Design review of the part built by this model. Coordinates are the model's own, in mm. A direction names the side the tool comes from. Coordinates: 2 decimals unless noted, no trailing zeros. Write each loop counter-clockwise with the first axis right and the second up, starting at its lowest first coordinate (ties: lowest second). Pieces come first, ordered by that corner, then holes. Notation, with made-up numbers: M 20.25,4 L 27.25,4 A26 cw 27.25,28 Z; hole C 72.5,-12.75 d10. An arc over 180 degrees is marked long. Return JSON: item names as keys, results as strings. Group by question number.
```python
from build123d import *

# Parameters (mm, degrees)
F0_R     = 2.25
F0_R_2   = 4
F1_DEPTH = 1.5


with BuildPart() as f1:
    # F0 (on Top) → F1 (new body)
    with BuildSketch(Plane.XY):
        Polygon((-7.522005, 11.843878), (-49.622005, 11.843878), (-49.622005, -3.456122), (-7.522005, -3.456122), (4.677995, -10.218692), (11.677995, -10.218692), (11.677995, 25.220647), (10.617335, 26.281308), (-7.522005, 26.281308), align=None)
        with Locations((-34.622005, 4.193878)):
            Circle(F0_R, mode=Mode.SUBTRACT)
        with Locations((-22.622005, 4.193878)):
            Circle(F0_R, mode=Mode.SUBTRACT)
        with Locations((2.177995, 5.281308)):
            Circle(F0_R_2, mode=Mode.SUBTRACT)
    extrude(amount=F1_DEPTH)


solid = f1.part
```
Item 1: The part is to be moulded in two halves that separate along Y. For faces 4 (the flat face through (2, 26.281, 1)), 5 (the cylindrical face through (-23.11, 1.997, 0.74)), 6 (the flat face through (11.678, 7, 1)), say which applies: pulls with the +Y half, pulls with the -Y half, needs draft (parallel to the pull), parting line crosses it, or undercut.
Item 2: Add section A-A (y = 3). Write out the cut boundary in (x, z).
Item 3: For line 1 (Y direction, x = -19.5, z = 0.6); line 2 (X direction, y = 20, z = 1.2); line 3 (X direction, y = 7.5, z = 0.8), list the stretches that pass through material, from the lowest coordinate up.
Item 4: Add section B-B (z = 0.75). Write out the cut boundary in (x, y).
Item 5: Machinability: for faces 1 (the flat face through (-29, -3.456, 1)), 2 (the flat face through (-28, 11.844, 1)), 3 (the flat face through (-13, 8, 1.5)), which of the approach directions +Z, -Z, +X, -X, +Y, -Y give a long, thin tool a straight path to every point of the face, cutting with its end or side? Answer none if there is none.
Item 6: For pin 1 (2.5 mm diameter, centred on x = -22.62, y = 4.19, fed in from -Z), flat-tipped, find the tip position at first contact; note if it passes through.
Item 7: Add section C-C (x = -40). Write out the cut boundary in (y, z), plus the area to 4 significant figures.
Item 8: Add section D-D (y = 20.5). Write out the cut boundary in (x, z), plus the area to 3 significant figures.
Geometry check:
{
 "1": {"face 4": "pulls with the +Y half", "face 5": "undercut", "face 6": "needs draft"},
 "2": {"outline": "M -49.62,0 L -36.53,0 L -36.53,1.5 L -49.62,1.5 Z; M -32.71,0 L -24.53,0 L -24.53,1.5 L -32.71,1.5 Z; M -20.71,0 L -1.11,0 L -1.11,1.5 L -20.71,1.5 Z; M 5.46,0 L 11.68,0 L 11.68,1.5 L 5.46,1.5 Z"},
 "3": {"line 1": "-3.46 to 11.84", "line 2": "-7.52 to 11.68", "line 3": "-49.62 to -1.15, 5.51 to 11.68"},
 "4": {"outline": "M -49.62,-3.46 L -7.52,-3.46 L 4.68,-10.22 L 11.68,-10.22 L 11.68,25.22 L 10.62,26.28 L -7.52,26.28 L -7.52,11.84 L -49.62,11.84 Z; hole C -34.62,4.19 d4.5; hole C -22.62,4.19 d4.5; hole C 2.18,5.28 d8"},
 "5": {"face 1": "+Z, -Z, -X, -Y", "face 2": "+Z, -Z, -X, +Y", "face 3": "+Z, +X, -X, +Y, -Y"},
 "6": {"pin 1": "through"},
 "7": {"outline": "M -3.46,0 L 11.84,0 L 11.84,1.5 L -3.46,1.5 Z", "area": "22.95 mm^2"},
 "8": {"outline": "M -7.52,0 L 11.68,0 L 11.68,1.5 L -7.52,1.5 Z", "area": "28.8 mm^2"}
}
